Check sheet for the modelled part. Datum: model origin and axes. Units: mm. A direction names the side the tool comes from. Round coordinates to 2 decimals unless told otherwise and drop trailing zeros. Write each loop counter-clockwise with the first axis right and the second up, starting at its lowest first coordinate (ties: lowest second). Pieces come first, ordered by that corner, then holes. Notation, with made-up numbers: (-11, 3) - (13, 3) arc R12 ccw to (13, 7) - close; hole circle Ø6 at (72.5, 1.5). An arc over 180 degrees is marked (long way). Answer as a JSON object with one key per item and string values. Group by question number.
Item 1: Set-up check for faces 1 (the flat face through (-7, -15, 3)), 2 (the flat face through (7, -30, 7)), 3 (the flat face through (-2.5, -7, 20)), 4 (the cylindrical face through (2.703, 9.86, 8.584)): record each of +Z, -Z, +X, -X, +Y, -Y from which the full face is reachable in a straight line by a thin tool's end or side.
Item 2: Thickness scan on line 1 (Y direction, x = 6, z = 10.16); line 2 (Y direction, x = 6.3, z = 0.16); line 3 (X direction, y = -25.5, z = -3.5). Record the ranges inside material, lowest first.
Item 3: Release check for a two-part mould opening along Z. For faces 5 (the cylindrical face through (5.528, -23.013, 0.355)), 6 (the flat face through (9.5, -12, 5)), 7 (the cylindrical face through (5.528, -23.235, 9.354)), 8 (the flat face through (-7, -21, -12.67)) record: pulls with the +Z half, pulls with the -Z half, needs draft (parallel to the pull), parting line crosses it, or undercut.
Item 4: Gauge pin test, flat ends, axial feed: P1, Ø2, axis at x = -8.5, y = -17.5, coming from the +Z side; P2, Ø11, axis at x = -11, y = -9.5, coming from the +Z side; P3, Ø3.5, axis at y = -24.5, z = 10.16, coming from the +X side. Record the tip position at first contact, or that the pin passes through.
Item 5: Sectioned sample at B-B on z = 10.16. Record the boundary of the cut face in (x, y).
Item 6: Sectioned sample at D-D on x = 5.25. Record the boundary of the cut face in (y, z).
Item 7: Sectioned sample at C-C on x = 0. Record the boundary of the cut face in (y, z), plus the area to 3 significant figures.
Item 8: Sectioned sample at A-A on y = -24.5. Record the boundary of the cut face in (x, z), plus the area to 3 significant figures.
```python
from build123d import *

# Parameters (mm, degrees)
SKETCH_1_R          = 9
EXTRUDE_1_DEPTH     = 20
SKETCH_2_W          = 20
SKETCH_2_H          = 43.67
EXTRUDE_2_DEPTH     = 15
SKETCH_3_W          = 14
SKETCH_3_H          = 15
CUT_EXTRUDE_1_DEPTH = 38.433273968
SKETCH_4_W          = 20
SKETCH_4_H          = 4
EXTRUDE_3_DEPTH     = 17.26
CUT_EXTRUDE_2_DEPTH = 50.193064552
EXTRUDE_4_DEPTH     = 30
SKETCH_7_R          = 1.5
CUT_EXTRUDE_3_DEPTH = 50.454095887
EXTRUDE_5_DEPTH     = 6
CHAMFER_1_SIZE      = 2


with BuildPart() as part:
    # Эскиз1 → Бобышка-Вытянуть1 (new body)
    with BuildSketch(Plane(origin=(0, 0, 0), x_dir=(1, 0, 0), z_dir=(0, 1, 0))):
        with Locations(Location((0, 0, 0), (0, 0, 270))):
            Circle(SKETCH_1_R)
    extrude(amount=EXTRUDE_1_DEPTH)

    # Эскиз2 → Бобышка-Вытянуть2 (add)
    with BuildSketch(Plane.XZ):
        with Locations((-6.5, 5.165)):
            Rectangle(SKETCH_2_W, SKETCH_2_H)
    extrude(amount=EXTRUDE_2_DEPTH)

    # Эскиз3 → Вырез-Вытянуть1 (cut, through all)
    with BuildSketch(Plane(origin=(0, 0, 0), x_dir=(1, 0, 0), z_dir=(0, 1, 0))):
        with Locations((-9.5, -19.5)):
            Rectangle(SKETCH_3_W, SKETCH_3_H)
    extrude(amount=-CUT_EXTRUDE_1_DEPTH, mode=Mode.SUBTRACT)

    # Эскиз4 → Бобышка-Вытянуть3 (add)
    with BuildSketch(Plane.XZ.offset(15)):
        with Locations((-6.5, -14.67)):
            Rectangle(SKETCH_4_W, SKETCH_4_H)
    extrude(amount=EXTRUDE_3_DEPTH)

    # Эскиз5 → Вырез-Вытянуть2 (cut, through all)
    with BuildSketch(Plane.ZY.offset(16.5)):
        Polygon((-12.67, -32.26), (-12.67, -28.031597138), (-16.67, -32.26), align=None)
    extrude(amount=-CUT_EXTRUDE_2_DEPTH, mode=Mode.SUBTRACT)

    # Эскиз6 → Бобышка-Вытянуть4 (add)
    with BuildSketch(Plane.XZ):
        Polygon((3.5, 8.291561976), (3.5, 27), (9.5, 27), (9.5, -16.67), (3.5, -16.67), (3.5, -8.291561976), align=None)
    extrude(amount=EXTRUDE_4_DEPTH)

    # Эскиз7 → Вырез-Вытянуть3 (cut, through all)
    with BuildSketch(Plane(origin=(9.5, 0, 0), x_dir=(0, 0, -1), z_dir=(1, 0, 0))):
        with Locations((-10.16, -24.5)):
            Circle(SKETCH_7_R)
        with Locations((-0.16, -24.5)):
            Circle(SKETCH_7_R)
    extrude(amount=-CUT_EXTRUDE_3_DEPTH, mode=Mode.SUBTRACT)

    # Эскиз8 → Бобышка-Вытянуть5 (add)
    with BuildSketch(Plane(origin=(3.5, 0, 0), x_dir=(0, 0, -1), z_dir=(1, 0, 0))):
        Polygon((16.67, -30), (14.532076937, -30), (16.67, -32.26), align=None)
    extrude(amount=EXTRUDE_5_DEPTH)

    # Фаска1
    chamfer_1_edges = [part.edges().sort_by_distance(p)[0] for p in [
        (9.5, -24.5, 11.66),
        (9.5, -24.5, 1.66),
    ]]
    chamfer(chamfer_1_edges, length=CHAMFER_1_SIZE)


solid = part.part
```
Completed:
{
 "1": {"face 1": "+Z, -X, -Y", "face 2": "+Z, +X, -X, -Y", "face 3": "+Z, -X, +Y, -Y", "face 4": "+Y"},
 "2": {"line 1": "-30 to -26, -23 to 0", "line 2": "-30 to -26, -23 to 20", "line 3": "3.5 to 9.5"},
 "3": {"face 5": "undercut", "face 6": "needs draft", "face 7": "undercut", "face 8": "pulls with the +Z half"},
 "4": {"P1": "z = -12.67", "P2": "z = 12", "P3": "x = 7.75"},
 "5": {"outline": "(-16.5, -15) - (3.5, -15) - (3.5, -23) - (7.5, -23) - (9.5, -21) - (9.5, 0) - (-16.5, 0) - close; (3.5, -30) - (9.5, -30) - (9.5, -28) - (7.5, -26) - (3.5, -26) - close"},
 "6": {"outline": "(-32.26, -16.67) - (0, -16.67) - (0, -7.31) - (20, -7.31) - (20, 7.31) - (0, 7.31) - (0, 27) - (-30, 27) - (-30, -14.53) - close; hole circle Ø3 at (-24.5, 0.16); hole circle Ø3 at (-24.5, 10.16)"},
 "7": {"outline": "(-32.26, -16.67) - (0, -16.67) - (0, -9) - (20, -9) - (20, 9) - (0, 9) - (0, 27) - (-15, 27) - (-15, -12.67) - (-28.03, -12.67) - close", "area": "1,080 mm²"},
 "8": {"outline": "(-16.5, -16.67) - (9.5, -16.67) - (9.5, -3.34) - (7.5, -1.34) - (3.5, -1.34) - (3.5, -12.67) - (-16.5, -12.67) - close; (3.5, 1.66) - (7.5, 1.66) - (9.5, 3.66) - (9.5, 6.66) - (7.5, 8.66) - (3.5, 8.66) - close; (3.5, 11.66) - (7.5, 11.66) - (9.5, 13.66) - (9.5, 27) - (3.5, 27) - close", "area": "298 mm²"}
}
